Part print with two shaded views. Sizes in mm from the minimum x, y, z corner. Give positions to 0.01 mm unless a question says otherwise; leave off trailing zeros. Loops run counter-clockwise (first coordinate to the right, second up) from the corner with the lowest first, then second, coordinate; pieces in that order, holes last. Notation, with made-up numbers: (80, 8) -> (129, 8) arc R16 ccw to (129, 23) -> close; hole circle Ø1 at (23, 69.25). An arc over 180 degrees is marked (long way). One line per question, with ' | ' between items. Start each with the question number.
(1) Slice it at B-B, the plane y = 2.75. Write the cut outline in (x, z), then the cut area to 3 significant figures.
(2) Slice it at A-A, the plane x = 8.8. Write the cut outline in (y, z).
(3) Slice it at C-C, the plane x = 4.8. Write the cut outline in (y, z).
(4) Flat gauge pins, fed straight in: pin 1 Ø4 at (x, y) = (9, 4.5) entering from +Z; pin 2 Ø2 at (x, y) = (2, 4) entering from -Z. Where does each tip first touch, or does it go through?
(5) Slice it at D-D, the plane y = 6. Write the cut outline in (x, z).
(6) Mould opens along X. For the marked faces 1, 2 and 3 say: pulls with the +X half, pulls with the -X half, needs draft (parallel to the pull), parting line crosses it, or undercut.
(7) Drill centre lines: L1, parallel to X at y = 4.5, z = 5.5 (1 decimal); L2, parallel to X at y = 1.5, z = 6.75 (1 decimal); L3, parallel to Z at x = 8.8, y = 5.1 (1 decimal). Where is each one in solid material? Low to high. Write a range as from..to.
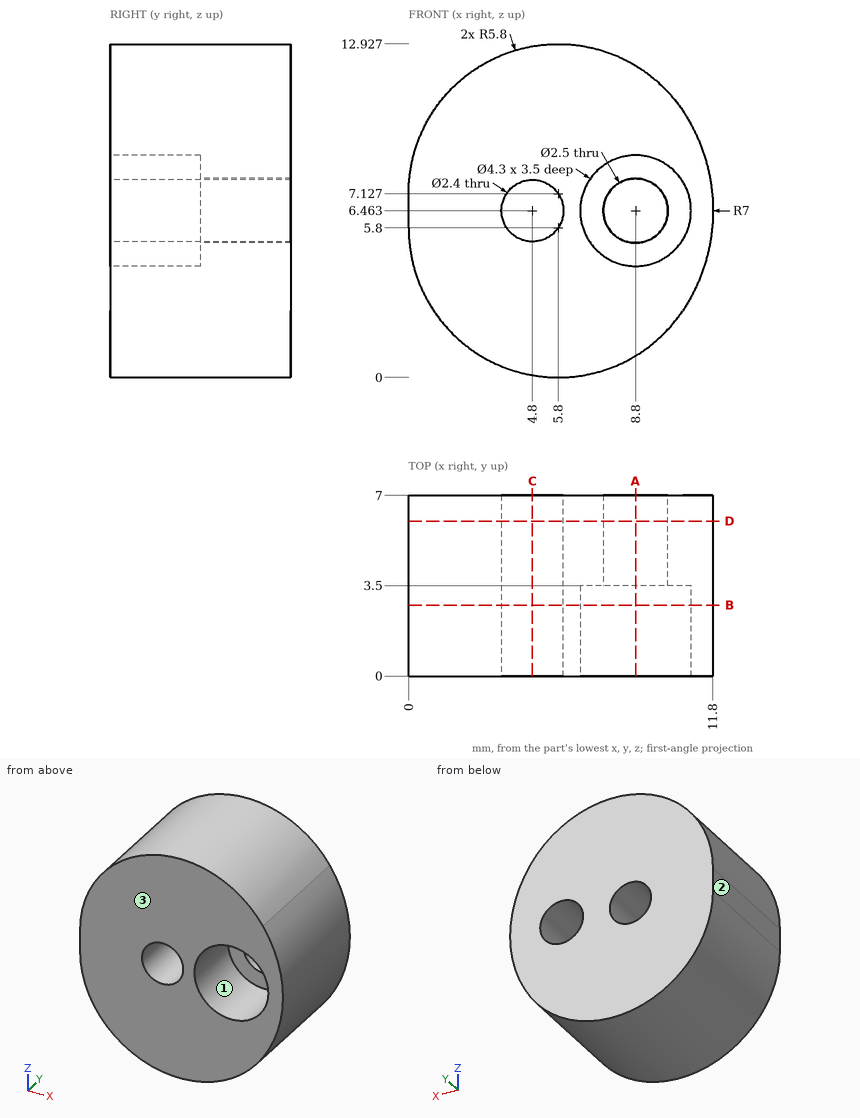
Final values:
1) outline: (0, 5.8) arc R5.8 ccw to (10.63, 2.59) arc R7 ccw to (10.63, 10.33) arc R5.8 ccw to (0, 7.13) -> close; hole circle Ø2.4 at (4.8, 6.46); hole circle Ø4.3 at (8.8, 6.46) | area: 103 mm2
2) outline: (0, 0.84) -> (7, 0.84) -> (7, 5.21) -> (3.5, 5.21) -> (3.5, 4.31) -> (0, 4.31) -> close; (0, 8.61) -> (3.5, 8.61) -> (3.5, 7.71) -> (7, 7.71) -> (7, 12.09) -> (0, 12.09) -> close
3) outline: (0, 0.09) -> (7, 0.09) -> (7, 5.26) -> (0, 5.26) -> close; (0, 7.66) -> (7, 7.66) -> (7, 12.84) -> (0, 12.84) -> close
4) pin 1: z = 12.8 | pin 2: z = 0.72
5) outline: (0, 5.8) arc R5.8 ccw to (10.63, 2.59) arc R7 ccw to (10.63, 10.33) arc R5.8 ccw to (0, 7.13) -> close; hole circle Ø2.4 at (4.8, 6.46); hole circle Ø2.5 at (8.8, 6.46)
6) face 1: undercut | face 2: pulls with the -X half | face 3: needs draft
7) L1: 0..4.1, 5.5..8, 9.6..11.7 | L2: 0..3.6, 6..6.7, 10.9..11.8 | L3: 0.8..5.2, 7.7..12.1
